Geometry: see drawing. Coordinates: mm, zero at the bounding-box minimum. A direction names the side the tool comes from. Give positions to 0.01 mm unless a question says otherwise; leave off trailing zeros. Loops run counter-clockwise (first coordinate to the right, second up) from the corner with the lowest first, then second, coordinate; pieces in that order, holes last. Notation, with made-up numbers: (-34, -19.5) - (10, -19.5) arc R27 ccw to (10, 0.5) - close; hole circle Ø5 at (30.25, -15.5). An arc over 180 degrees is marked (long way). Use one line per item in the form item = value.
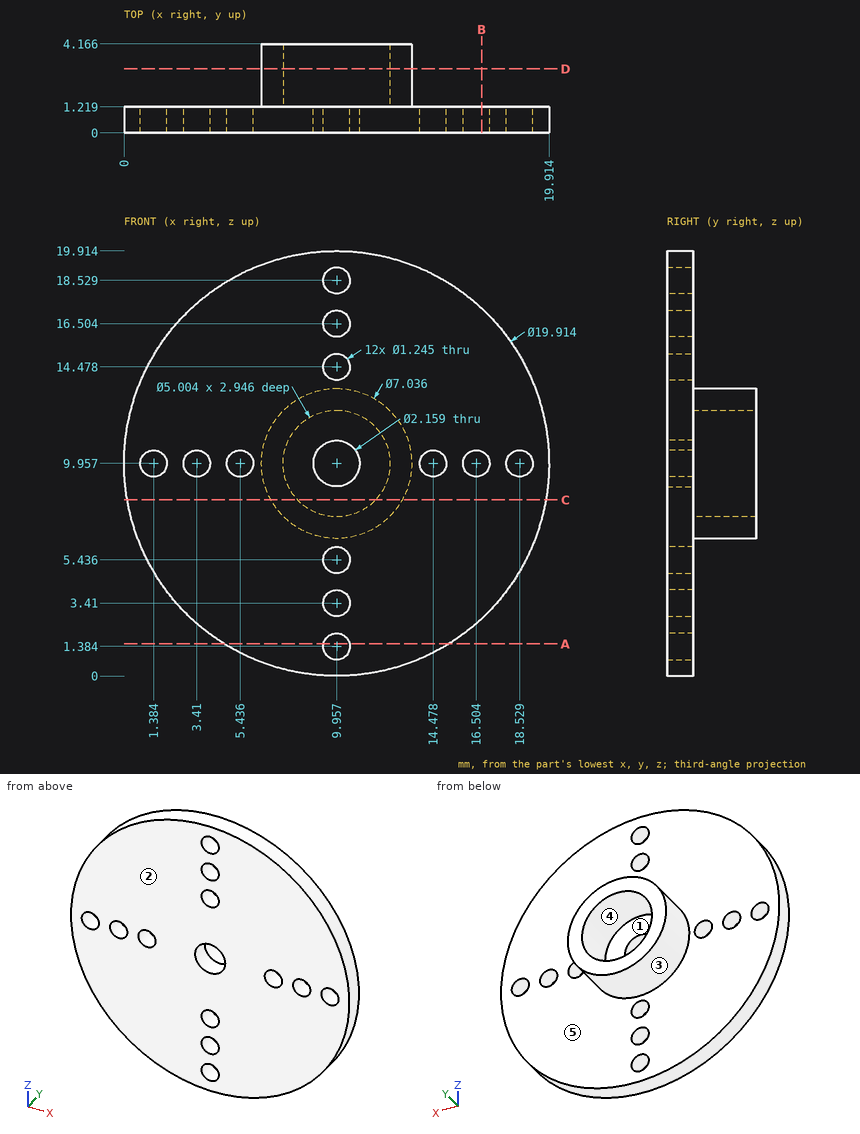
(1) Cut plane C-C (z = 8.25). Return the cut outline in (x, y) (1 decimal).
Solution:
outline = (0.1, 0) - (19.8, 0) - (19.8, 1.2) - (13, 1.2) - (13, 4.2) - (11.8, 4.2) - (11.8, 1.2) - (8.1, 1.2) - (8.1, 4.2) - (6.9, 4.2) - (6.9, 1.2) - (0.1, 1.2) - close
(2) Cut plane D-D (y = 3). Return the cut outline in (x, z) (1 decimal).
Solution:
outline = circle Ø7 at (10, 10); hole circle Ø5 at (10, 10)
(3) Access query for the marked faces 1 and 2. Directions: +Z, -Z, +X, -X, +Y, -Y. A direction counts if a zero-diameter tool reaches every point of the face in a straight line with its end or side. Return the directions, or none.
Solution:
face_1 = +Y
face_2 = +Z, -Z, +X, -X, -Y
(4) Pull-direction query (Z, two-part tool) for the marked faces 3, 4 and 5; classes: released by +Z, released by -Z, zero draft, split by the parting line, or undercut.
Solution:
face_3 = split by the parting line
face_4 = undercut
face_5 = zero draft
(5) Pin query (flat end, axial travel): P1, Ø1.5, axis at x = 10, z = 11, coming from the +Y side; P2, Ø1, axis at x = 11.5, y = 1, coming from the -Z side (1 decimal); P3, Ø1, axis at y = 1, z = 17, coming from the -X side. Return the tip coordinate at first contact, or that it passes through.
Solution:
P1 = 1.22
P2 = 0.1
P3 = 2.45
(6) Cut plane B-B (x = 16.75). Return the cut outline in (y, z) (1 decimal).
Solution:
outline = (0, 2.7) - (1.2, 2.7) - (1.2, 9.4) - (0, 9.4) - close; (0, 10.5) - (1.2, 10.5) - (1.2, 17.2) - (0, 17.2) - close
(7) Material intervals for L1, parallel to Y at x = 9, z = 14.25; L2, parallel to Z at x = 11, y = 3 (1 decimal); L3, parallel to Z at x = 18.75, y = 0.5 (1 decimal), sorted ascending. Write a range as from..to.
Solution:
L1 = 0..1.22
L2 = 6.6..7.7, 12.2..13.3
L3 = 5.3..9.4, 10.5..14.6
(8) Cut plane A-A (z = 1.5). Return the cut outline in (x, y) (1 decimal), plus the area to 3 significant figures.
Solution:
outline = (4.7, 0) - (9.3, 0) - (9.3, 1.2) - (4.7, 1.2) - close; (10.6, 0) - (15.2, 0) - (15.2, 1.2) - (10.6, 1.2) - close
area = 11.3 mm2
